```python
from build123d import *

# Parameters (mm, degrees)
F0_W     = 25.4
F0_H     = 25.4
F1_DEPTH = 25.4
F2_SIZE2 = 25.39999
F2_SIZE  = 12.69999


# Not quite as in the source:
# - a fillet or chamfer is up to 0.001 mm smaller than in the source, because OpenCascade refuses the exact size


with BuildPart() as f1:
    # F0 (on Front) → F1 (new body)
    with BuildSketch(Plane.XZ):
        with Locations((12.7, 12.7)):
            Rectangle(F0_W, F0_H)
    extrude(amount=F1_DEPTH)

    # F2 (size 12.7 and 25.4 in the source; OpenCascade refuses exactly that, so slightly less here)
    f2_edges = [f1.edges().sort_by_distance(p)[0] for p in [
        (25.4, -12.7, 25.4),
        (0, -12.7, 25.4),
        (12.7, 0, 25.4),
        (12.7, -25.4, 25.4),
    ]]
    f2_side = f1.faces().sort_by_distance((12.7, -12.7, 25.4))[0]
    chamfer(f2_edges, length=F2_SIZE, length2=F2_SIZE2, reference=f2_side)


solid = f1.part
```
Input: part model. Units: mm. Frame: model coordinates. Round coordinates to 2 decimals unless told otherwise and drop trailing zeros. Loops run counter-clockwise (first coordinate to the right, second up) from the corner with the lowest first, then second, coordinate; pieces in that order, holes last. Notation, with made-up numbers: (15.5, 79) - (51.5, 79) arc R17 ccw to (51.5, 97) - close; hole circle Ø3 at (52.25, 12.25). An arc over 180 degrees is marked (long way). One line per item, written item: value. Start each with the question number.
(1) Section C-C, the plane z = 3. Return loops of the section in (x, y), plus the area to 3 significant figures.
(2) Contact query for flat-ended pins moving along their axis: P1, Ø12, axis at y = -7, z = 22.5, coming from the +X side; P2, Ø10, axis at y = -19.5, z = 8.5, coming from the +X side; P3, Ø10, axis at x = 19.5, z = 9.5, coming from the -Y side; P4, Ø5, axis at x = 7, z = 20, coming from the +Y side. Output: stop coordinate, or through.
(3) Ray query, line 1 (Y direction, x = 11.5, z = 21.25) (3 decimals); line 2 (Z direction, x = 18.25, y = -21.25); line 3 (X direction, y = -15.75, z = 15.75) (3 decimals). Return the intervals inside material, ascending. Write a range as [from, to].
Results below:
1. outline: (1.5, -23.9) - (23.9, -23.9) - (23.9, -1.5) - (1.5, -1.5) - close
1. area: 502 mm^2
2. P1: x = 17.08
2. P2: x = 23.65
2. P3: y = -23.15
2. P4: through
3. line 1: [-14.775, -10.625]
3. line 2: [0, 8.3]
3. line 3: [7.875, 17.525]
